from build123d import *
from OCP.BRepFilletAPI import BRepFilletAPI_MakeChamfer

# Parameters (mm, degrees)
SKETCH1_R           = 7.5
BOSS_EXTRUDE1_DEPTH = 10
SKETCH2_R           = 15.403290795
BOSS_EXTRUDE2_DEPTH = 7
SKETCH4_R           = 6.56
CUT_EXTRUDE1_DEPTH  = 5
CHAMFER1_SIZE       = 8
CHAMFER2_SIZE       = 0.3
CHAMFER2_SIZE2      = 0.824243226


with BuildPart() as part:
    # Sketch1 → Boss-Extrude1 (new body)
    with BuildSketch(Plane.XY):
        Circle(SKETCH1_R)
        with BuildLine():
            Line((-2.6, -1.778341924), (-2.6, 1.778341924))
            ThreePointArc((-2.6, 1.778341924), (3.15, 0), (-2.6, -1.778341924))
        make_face(mode=Mode.SUBTRACT)
    extrude(amount=BOSS_EXTRUDE1_DEPTH)

    # Sketch2 → Boss-Extrude2 (add)
    with BuildSketch(Plane.XY):
        Circle(SKETCH2_R)
    extrude(amount=-BOSS_EXTRUDE2_DEPTH)

    # Sketch4 → Cut-Extrude1 (cut)
    with BuildSketch(Plane(origin=(0, 0, -7), x_dir=(-1, 0, 0), z_dir=(0, 0, -1))):
        with Locations((0, 5)):
            Circle(SKETCH4_R)
    extrude(amount=-CUT_EXTRUDE1_DEPTH, mode=Mode.SUBTRACT)

    # Chamfer1
    # the kernel refuses this chamfer: 8 mm, written as the material it adds along each edge
    with BuildSketch(Plane(origin=(0, 0, 0), x_dir=(1, 0, 0), z_dir=(0, -1, 0))) as chamfer1_piece_1_section:
        Polygon((7.5 + CHAMFER1_SIZE, 0), (7.5, CHAMFER1_SIZE), (7.5, 0), align=None)
    chamfer1_piece_1 = revolve(axis=Axis((0, 0, 0), (0, 0, 1)), mode=Mode.PRIVATE)
    chamfer1_piece_1 = chamfer1_piece_1 & Plane(origin=(0, 0, 4.06906202), x_dir=(1, 0, 0), z_dir=(0, 0, 1)) * Cylinder(15.403290795, 62, mode=Mode.PRIVATE)
    add(chamfer1_piece_1)

    # Chamfer2: one chamfer whose edges measure the first distance from different faces: ONE call of the kernel's chamfer builder (chamfer() names one face for all edges)
    chamfer2_edges_1 = [part.edges().sort_by_distance(p)[0] for p in [
        (6.56, 5, -7),
    ]]
    chamfer2_side_1 = [part.faces().sort_by_distance(p)[0] for p in [
        (-14.96761994, 0, -7),
    ]]
    chamfer2_edges_2 = [part.edges().sort_by_distance(p)[0] for p in [
        (3.15, 0, 10),
        (-2.6, 0, 10),
    ]]
    chamfer2_side_2 = [part.faces().sort_by_distance(p)[0] for p in [
        (-7.287867966, 0, 10),
    ]]
    chamfer2 = BRepFilletAPI_MakeChamfer(part.part.solid().wrapped)
    for e in chamfer2_edges_1:
        chamfer2.Add(CHAMFER2_SIZE, CHAMFER2_SIZE2, e.wrapped, chamfer2_side_1[0].wrapped)  # the first distance lies on this face
    for e in chamfer2_edges_2:
        chamfer2.Add(CHAMFER2_SIZE, CHAMFER2_SIZE2, e.wrapped, chamfer2_side_2[0].wrapped)  # the first distance lies on this face
    add(Compound.cast(chamfer2.Shape()), mode=Mode.REPLACE)


solid = part.part
The listing builds one solid part. Answer for the finished solid, in the listing's coordinates (mm). A direction names the side the tool comes from. Coordinates: 2 decimals unless noted, no trailing zeros. Loops run counter-clockwise (first coordinate to the right, second up) from the corner with the lowest first, then second, coordinate; pieces in that order, holes last. Notation, with made-up numbers: (-38.75, 16) -> (-13.75, 16) arc R14 ccw to (-13.75, 30) -> close; hole circle Ø7 at (41.25, -32.5). An arc over 180 degrees is marked (long way). Answer in a Markdown table with one row per item. Add a question column.
1. Consider line 1 (Y direction, x = 0, z = -4.85); line 2 (Z direction, x = 4, y = 4); line 3 (X direction, y = 0, z = 6.5). Determine where each line is inside the solid, lowest interval first. Write a range as [from, to].
2. For faces 1 (the flat face through (0, -3, -7)), 2 (the flat face through (0, 0, 0)), 3 (the flat face through (0, 5, -2)), determine the directions among +Z, -Z, +X, -X, +Y, -Y from which every point of the face is accessible in a straight line to the end or side of a thin tool.
3. The part is cut by section A-A, the plane z = 4. Write down the section's boundary in (x, y), then the cut area to 3 significant figures.
4. Determine the mould class of faces 4 (the cylindrical face through (-7.493, 0.33, 8.986)), 5 (the flat face through (2, -3, 10)), 6 (the conical face through (3.23, 0.12, 9.4)) for opening direction Y: +Y half, -Y half, draft (parallel to the pull), parting line (faces both ways), or undercut.
5. The part is cut by section C-C, the plane z = -1. Write down the section's boundary in (x, y).
6. Flat-ended cylindrical pins translate along their axes: P1, Ø4, axis at y = 0, z = 8, coming from the -X side; P2, Ø1.5, axis at x = 9, z = -1.5, coming from the -Y side; P3, Ø4, axis at y = 0.5, z = 3, coming from the +X side. Find the tip coordinate at first contact, or state that the pin passes through.
7. The part is cut by section B-B, the plane x = 0. Write down the section's boundary in (y, z).
8. The part is cut by section D-D, the plane z = -4.75. Write down the section's boundary in (x, y).
Answer below:
| question | item | result |
|---|---|---|
| 1 | line 1 | [-15.4, -1.56], [11.56, 15.4] |
| 1 | line 2 | [-2, 10] |
| 1 | line 3 | [-9, -2.6], [3.15, 9] |
| 2 | face 1 | -Z, +X, -X, +Y, -Y |
| 2 | face 2 | +Z |
| 2 | face 3 | -Z |
| 3 | outline | circle Ø23 at (0, 0); hole (-2.6, -1.78) arc R3.15 ccw (long way) to (-2.6, 1.78) -> close |
| 3 | area | 386 mm2 |
| 4 | face 4 | parting line |
| 4 | face 5 | draft |
| 4 | face 6 | undercut |
| 5 | outline | circle Ø30.81 at (0, 0) |
| 6 | P1 | x = -9.5 |
| 6 | P2 | y = -13.01 |
| 6 | P3 | x = 14.49 |
| 7 | outline | (-15.4, -7) -> (-1.86, -7) -> (-1.56, -6.18) -> (-1.56, -2) -> (11.56, -2) -> (11.56, -6.18) -> (11.86, -7) -> (15.4, -7) -> (15.4, 0.1) -> (7.5, 8) -> (7.5, 10) -> (3.45, 10) -> (3.15, 9.18) -> (3.15, 0) -> (-3.15, 0) -> (-3.15, 9.18) -> (-3.45, 10) -> (-7.5, 10) -> (-7.5, 8) -> (-15.4, 0.1) -> close |
| 8 | outline | circle Ø30.81 at (0, 0); hole circle Ø13.12 at (0, 5) |
